Part print with two shaded views. Sizes in mm from the minimum x, y, z corner. Coordinates: 2 decimals unless noted, no trailing zeros. Write each loop counter-clockwise with the first axis right and the second up, starting at its lowest first coordinate (ties: lowest second). Pieces come first, ordered by that corner, then holes. Notation, with made-up numbers: (-31, -40) - (2, -40) arc R16 ccw to (2, -9) - close; hole circle Ø3 at (50, 75). An arc over 180 degrees is marked (long way). One line per question, with ' | ' between items. Start each with the question number.
1. Band-saw the part on B-B, the plane y = 0.95. Write the cut outline in (x, z), then the cut area to 3 significant figures.
2. Flat gauge pins, fed straight in: P1, Ø2.5, axis at x = 90, z = 27.5, coming from the -Y side; P2, Ø1, axis at x = 73.5, y = 2.5, coming from the -Z side. Where does each tip first touch, or does it go through?
3. Band-saw the part on A-A, the plane x = 50. Write the cut outline in (y, z), then the cut area to 3 significant figures.
4. Band-saw the part on D-D, the plane z = 27.5. Write the cut outline in (x, y).
5. Probe line 1 (X direction, y = 1.6, z = 50); line 2 (X direction, y = 0.95, z = 27.5); line 3 (Z direction, x = 90, y = 0.8). List the from-to ranges inside material, lowest first.
6. Band-saw the part on C-C, the plane z = 50. Write the cut outline in (x, y).
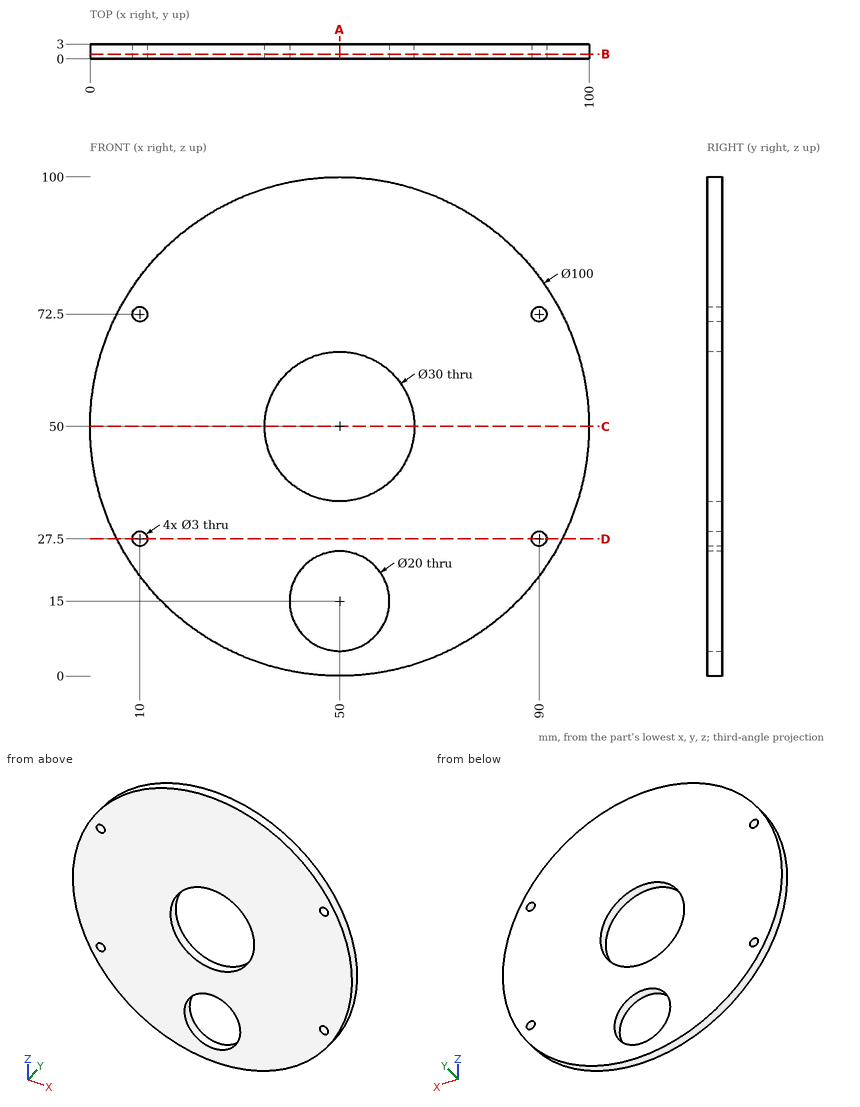
Filled in:
1) outline: circle Ø100 at (50, 50); hole circle Ø3 at (10, 27.5); hole circle Ø3 at (10, 72.5); hole circle Ø30 at (50, 50); hole circle Ø20 at (50, 15); hole circle Ø3 at (90, 27.5); hole circle Ø3 at (90, 72.5) | area: 6,800 mm²
2) P1: passes through | P2: stops at z = 5.6
3) outline: (0, 0) - (3, 0) - (3, 5) - (0, 5) - close; (0, 25) - (3, 25) - (3, 35) - (0, 35) - close; (0, 65) - (3, 65) - (3, 100) - (0, 100) - close | area: 150 mm²
4) outline: (5.35, 0) - (8.5, 0) - (8.5, 3) - (5.35, 3) - close; (11.5, 0) - (88.5, 0) - (88.5, 3) - (11.5, 3) - close; (91.5, 0) - (94.65, 0) - (94.65, 3) - (91.5, 3) - close
5) line 1: x = 0 to 35, 65 to 100 | line 2: x = 5.35 to 8.5, 11.5 to 88.5, 91.5 to 94.65 | line 3: z = 20 to 26, 29 to 71, 74 to 80
6) outline: (0, 0) - (35, 0) - (35, 3) - (0, 3) - close; (65, 0) - (100, 0) - (100, 3) - (65, 3) - close
